Design review of the part shown in the three views and the two pictorial views. Dimensions are in mm from the part's minimum x, y and z. Give positions to 0.01 mm unless a question says otherwise; leave off trailing zeros. Loops run counter-clockwise (first coordinate to the right, second up) from the corner with the lowest first, then second, coordinate; pieces in that order, holes last. Notation, with made-up numbers: (-3, 32) - (39, 32) arc R24 cw to (39, 54) - close; hole circle Ø1 at (47, -4.5). An arc over 180 degrees is marked (long way). Use CSV: the item, a comma, the result in double quotes. Start each with the question number.
1. Take a section at A-A on z = 101.6. Give the boundary of the cut face in (x, y), plus the area to 3 significant figures.
2. Wall thickness on line 1 (Z direction, x = 101.6, y = 4.5); line 2 (X direction, y = 3, z = 101.6); line 3 (X direction, y = 1, z = 174.5) (1 decimal): over which ranges is each line inside the solid? List them lowest first.
3. For pin 1 (1 mm diameter, centred on x = 156, y = 2.5, fed in from -Z) (1 decimal); pin 2 (2 mm diameter, centred on x = 168, y = 4, fed in from -Z); pin 3 (1.9 mm diameter, centred on y = 2, z = 176, fed in from +X); pin 4 (1.9 mm diameter, centred on x = 101.5, y = 4, fed in from -Z), all flat-tipped, find the tip position at first contact; note any pin that passes through.
4. Take a section at C-C on x = 101.6. Give the boundary of the cut face in (y, z), plus the area to 3 significant figures.
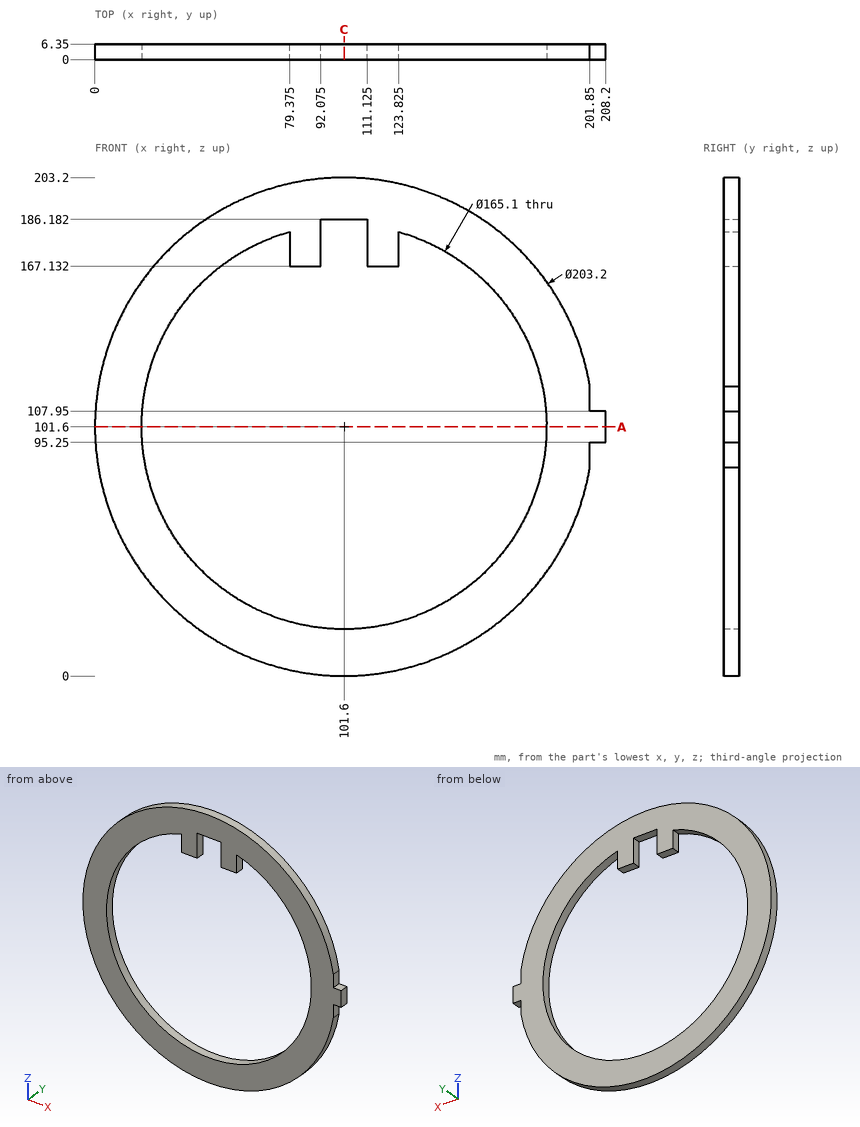
Check result:
1,outline,"(0, 0) - (19.05, 0) - (19.05, 6.35) - (0, 6.35) - close; (184.15, 0) - (208.2, 0) - (208.2, 6.35) - (184.15, 6.35) - close"
1,area,"274 mm²"
2,line 1,"z = 0 to 19.05, 186.18 to 203.2"
2,line 2,"x = 0 to 19.05, 184.15 to 208.2"
2,line 3,"x = 30.8 to 62.9, 79.4 to 92.1, 111.1 to 123.8, 140.3 to 172.4"
3,pin 1,"stops at z = 15.5"
3,pin 2,"stops at z = 23.85"
3,pin 3,"stops at x = 171.8"
3,pin 4,"stops at z = 0"
4,outline,"(0, 0) - (6.35, 0) - (6.35, 19.05) - (0, 19.05) - close; (0, 186.18) - (6.35, 186.18) - (6.35, 203.2) - (0, 203.2) - close"
4,area,"229 mm²"
